Read the model definition and answer for the solid it produces. Units are mm, in the model's axes. A direction names the side the tool comes from. Give positions to 0.01 mm unless a question says otherwise; leave off trailing zeros. Order: outer loops, then holes, each group sorted by start corner. A loop starts at its lowest first (then second) coordinate and runs counter-clockwise, first axis right, second up.
```python
from build123d import *

# Parameters (mm, degrees)
F1_DEPTH = 8
F2_R     = 13


with BuildPart() as f1:
    # F0 (on Top) → F1 (new body)
    with BuildSketch(Plane.XY):
        with BuildLine():
            Line((-11, 0), (-5.240036, 0))
            ThreePointArc((-5.240036, 0), (8.322113, 5.75), (-5.240036, 11.5))
            Line((-5.240036, 11.5), (-11, 11.5))
            Line((-11, 11.5), (-11, 9))
            Line((-11, 9), (-2.5, 9))
            Line((-2.5, 9), (-2.5, 2.5))
            Line((-2.5, 2.5), (-11, 2.5))
            Line((-11, 2.5), (-11, 0))
        make_face()
    extrude(amount=F1_DEPTH)

    # F2
    f2_edges = [f1.edges().sort_by_distance(p)[0] for p in [
        (-5.240036, 0, 4),
        (-5.240036, 11.5, 4),
    ]]
    fillet(f2_edges, radius=F2_R)


solid = f1.part
```
1) For a pull along X with two mould halves and no side action, classify faces 4 (the face through (8.32, 5.52, 3.94)), 5 (the face through (-6.085, 11.863, 4.056)), 6 (the face through (-10, 0, 4)) as released by +X, released by -X, zero draft, split by the parting line, or undercut.
Final values:
face 4: split by the parting line
face 5: released by -X
face 6: zero draft
2) A tool of negligible diameter and unlimited length cuts with its end or side. For faces 1 (the face through (-10, 11.5, 4)), 2 (the face through (-11, 1, 4)), 3 (the face through (-7, 2.5, 4)), from which of +Z, -Z, +X, -X, +Y, -Y can it reach the whole face along a straight path? Write none if from no direction.
Final values:
face 1: +Z, -Z, -X, +Y
face 2: +Z, -Z, -X, +Y, -Y
face 3: +Z, -Z, -X
3) The part is cut by section D-D on x = -7.5. Determine the outline of the cut face in (y, z), and give its area (3 significant figures).
Final values:
outline: (-0.1, 0) - (2.5, 0) - (2.5, 8) - (-0.1, 8) - close; (9, 0) - (11.6, 0) - (11.6, 8) - (9, 8) - close
area: 41.7 mm2
4) Given pin 1 (0.6 mm diameter, centred on x = -10.5, z = 2.5, fed in from +Y); pin 2 (2.5 mm diameter, centred on x = -5.5, z = 3.5, fed in from -Y); pin 3 (2 mm diameter, centred on x = 2, z = 4.5, fed in from -Y), each flat-ended and moving along its own axis, determine where each tip first touches the part or whether it passes through.
Final values:
pin 1: stops at y = 11.5
pin 2: stops at y = -0.95
pin 3: stops at y = -2.22
5) The part is cut by section C-C on y = 5.75. Determine the outline of the cut face in (x, z).
Final values:
outline: (-2.5, 0) - (8.32, 0) - (8.32, 8) - (-2.5, 8) - close
6) Consider L1, parallel to Y at x = -10, z = 3.5; L2, parallel to Y at x = -6.5, z = 1.25; L3, parallel to Y at x = 0, z = 6.5. Determine where each line is inside the solid, lowest interval first.
Final values:
L1: y = 0 to 2.5, 9 to 11.5
L2: y = -0.27 to 2.5, 9 to 11.77
L3: y = -2.24 to 13.74
7) The part is cut by section A-A on x = -9.5. Determine the outline of the cut face in (y, z), and give its area (3 significant figures).
Final values:
outline: (0, 0) - (2.5, 0) - (2.5, 8) - (0, 8) - close; (9, 0) - (11.5, 0) - (11.5, 8) - (9, 8) - close
area: 40.0 mm2
8) The part is cut by section B-B on z = 1.75. Determine the outline of the cut face in (x, y).
Final values:
outline: (-11, 0) - (-9.14, 0) arc R13 cw to (-3.28, -1.39) arc R8 ccw (long way) to (-3.28, 12.89) arc R13 cw to (-9.14, 11.5) - (-11, 11.5) - (-11, 9) - (-2.5, 9) - (-2.5, 2.5) - (-11, 2.5) - close
